```python
from build123d import *

# Parameters (mm, degrees)
F1_DEPTH = 3


with BuildPart() as f1:
    # F0 (on Front) → F1 (new body)
    with BuildSketch(Plane.XZ):
        Polygon((16, 56), (3, 56), (3, 42), (0, 42), (0, 28), (3, 28), (3, 14), (0, 14), (0, 0), (3, 0), (3, -14), (0, -14), (-10, -14), (-10, -17), (-20, -17), (-20, -14), (-30, -14), (-30, -17), (-40, -17), (-40, -14), (-47, -14), (-47, -20.5), (-50, -20.5), (-50, -27.5), (-47, -27.5), (-47, -34), (-33, -34), (-33, -31.112283), (-16, -31.112283), (-16, -34), (1, -34), (1, -31.112283), (18, -31.112283), (18, -34), (35, -34), (35, -31.112283), (52, -31.112283), (52, -34), (71, -34), (71, -16), (68, -16), (68, 2), (71, 2), (71, 20), (68, 20), (68, 38), (71, 38), (71, 56), (55, 56), (55, 53), (42, 53), (42, 56), (29, 56), (29, 53), (16, 53), align=None)
    extrude(amount=F1_DEPTH)


solid = f1.part
```
Source: CAD feature listing. Evaluate the final solid. Frame: model axes, mm. A direction names the side the tool comes from. Coordinates: 2 decimals unless noted, no trailing zeros. Loops run counter-clockwise (first coordinate to the right, second up) from the corner with the lowest first, then second, coordinate; pieces in that order, holes last. Notation, with made-up numbers: M -35.75,-6.5 L -9.75,-6.5 A19 ccw -9.75,20.5 Z; hole C -19.5,-8.5 d5. An arc over 180 degrees is marked long. Use a Markdown table: item, result. Add a question column.
Q1. Material intervals for L1, parallel to Z at x = 2.5, y = -2.35; L2, parallel to X at y = -2.4, z = 52; L3, parallel to Z at x = 26.5, y = -0.95, sorted ascending.
Q2. First-contact query: pin 1 (1.5 mm diameter, centred on x = -15.5, y = -1.5, fed in from +Z); pin 2 (1.5 mm diameter, centred on y = -2, z = -16, fed in from -X); pin 3 (1.5 mm diameter, centred on x = 49, y = -2, fed in from +Z). Flat tips, straight axial feed; report the tip coordinate or a pass-through.
Q3. Access query for faces 5 (the flat face through (55, -1, 55)), 6 (the flat face through (3, -1, 49)), 7 (the flat face through (35, -1, -33)), 8 (the flat face through (69, -1, 38)). Directions: +Z, -Z, +X, -X, +Y, -Y. A direction counts if a zero-diameter tool reaches every point of the face in a straight line with its end or side. Return the directions, or none.
Q4. Section query A-A, the plane x = 14. Return loops of the section in (y, z), and give its area (3 significant figures).
Q5. Draft query along X for faces 1 (the flat face through (3, -1, 21)), 2 (the flat face through (-16, -1, -33)), 3 (the flat face through (-25, -1, -14)), 4 (the flat face through (71, -1, 47)). Return one class per face: pulls with the +X half, pulls with the -X half, needs draft (parallel to the pull), parting line crosses it, or undercut.
Q6. Section query B-B, the plane z = 8. Return loops of the section in (x, y).
Result:
| question | item | result |
|---|---|---|
| 1 | L1 | z = -31.11 to -14, 0 to 14, 28 to 42 |
| 1 | L2 | x = 3 to 71 |
| 1 | L3 | z = -34 to 53 |
| 2 | pin 1 | stops at z = -17 |
| 2 | pin 2 | stops at x = -47 |
| 2 | pin 3 | stops at z = 53 |
| 3 | face 5 | +Z, +Y, -Y |
| 3 | face 6 | +Z, -X, +Y, -Y |
| 3 | face 7 | -Z, +Y, -Y |
| 3 | face 8 | +X, +Y, -Y |
| 4 | outline | M -3,-31.11 L 0,-31.11 L 0,56 L -3,56 Z |
| 4 | area | 261 mm2 |
| 5 | face 1 | pulls with the -X half |
| 5 | face 2 | undercut |
| 5 | face 3 | needs draft |
| 5 | face 4 | pulls with the +X half |
| 6 | outline | M 0,-3 L 71,-3 L 71,0 L 0,0 Z |
